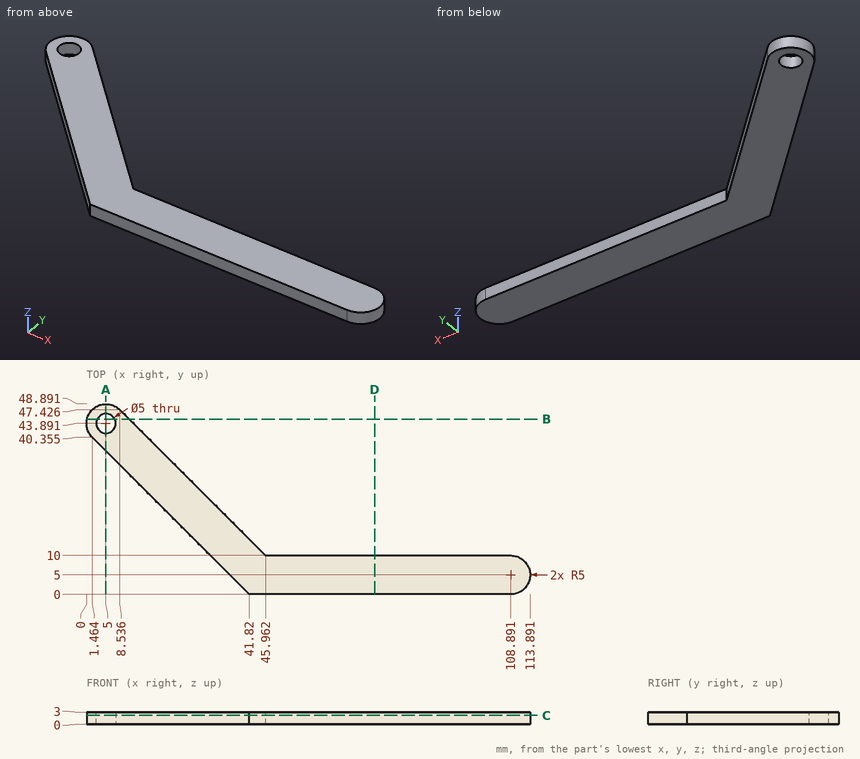
Geometry: see drawing. Coordinates: mm, zero at the bounding-box minimum. Coordinates: 2 decimals unless noted, no trailing zeros. Write each loop counter-clockwise with the first axis right and the second up, starting at its lowest first coordinate (ties: lowest second). Pieces come first, ordered by that corner, then holes. Notation, with made-up numbers: M 9.25,22.5 L 63.25,22.5 A24 ccw 63.25,42.5 Z; hole C 64.25,54.5 d3. An arc over 180 degrees is marked long. Use CSV: the item, a comma, the result in double quotes. Start each with the question number.
1. First-contact query: P1, Ø1, axis at x = 17.5, z = 1.5, coming from the -Y side; P2, Ø1.5, axis at x = 44.5, z = 2, coming from the +Y side. Flat tips, straight axial feed; report the tip coordinate or a pass-through.
2. Cut plane B-B on y = 45. Return the cut outline in (x, z) (1 decimal).
3. Cut plane A-A on x = 5. Return the cut outline in (y, z).
4. Cut plane D-D on x = 74. Return the cut outline in (y, z).
5. Ray query, probe 1 along Y at (x, z) = (82.5, 1.95); probe 2 along Y at (x, z) = (5, 1.7); probe 3 along X at (y, z) = (4, 0.85). Return the intervals inside material, ascending.
6. Cut plane C-C on z = 2.25. Return the cut outline in (x, y) (1 decimal).
Entries:
1,P1,"y = 23.82"
1,P2,"y = 12.21"
2,outline,"M 0.1,0 L 2.8,0 L 2.8,3 L 0.1,3 Z; M 7.2,0 L 11,0 L 11,3 L 7.2,3 Z"
3,outline,"M 36.82,0 L 41.39,0 L 41.39,3 L 36.82,3 Z; M 46.39,0 L 48.89,0 L 48.89,3 L 46.39,3 Z"
4,outline,"M 0,0 L 10,0 L 10,3 L 0,3 Z"
5,probe 1,"0 to 10"
5,probe 2,"36.82 to 41.39, 46.39 to 48.89"
5,probe 3,"37.82 to 113.79"
6,outline,"M 1.5,40.4 L 41.8,0 L 108.9,0 A5 ccw 108.9,10 L 46,10 L 8.5,47.4 A5 ccw Z; hole C 5,43.9 d5"
